from build123d import *

# Parameters (mm, degrees)
F0_R     = 1.6
F1_DEPTH = 2.3
F2_R     = 5.5
F3_DEPTH = 7.7
F5_DEPTH = 26.3
F6_R     = 1
F7_DEPTH = 5.55


with BuildPart() as f1:
    # F0 (on Top) → F1 (new body)
    with BuildSketch(Plane.XY):
        with BuildLine():
            Line((3, 5.765), (-3, 5.765))
            Line((-3, 5.765), (-10.043565, 3.861473))
            ThreePointArc((-10.043565, 3.861473), (-13, 0), (-10.043565, -3.861473))
            Line((-10.043565, -3.861473), (-3, -5.765))
            Line((-3, -5.765), (3, -5.765))
            Line((3, -5.765), (10.043565, -3.861473))
            ThreePointArc((10.043565, -3.861473), (13, 0), (10.043565, 3.861473))
            Line((10.043565, 3.861473), (3, 5.765))
        make_face()
        with Locations((-9, 0)):
            Circle(F0_R, mode=Mode.SUBTRACT)
        with Locations((9, 0)):
            Circle(F0_R, mode=Mode.SUBTRACT)
    extrude(amount=-F1_DEPTH)

    # F2 (on face) → F3 (join)
    with BuildSketch(Plane(origin=(0, 0, -2.3), x_dir=(1, 0, 0), z_dir=(0, 0, -1))):
        Circle(F2_R)
    extrude(amount=F3_DEPTH)

    # F4 (on face) → F5 (join)
    with BuildSketch(Plane(origin=(0, 0, -10), x_dir=(1, 0, 0), z_dir=(0, 0, -1))):
        with BuildLine():
            Line((4, 5.765), (-4, 5.765))
            ThreePointArc((-4, 5.765), (-6.5, 0), (-4, -5.765))
            Line((-4, -5.765), (4, -5.765))
            ThreePointArc((4, -5.765), (6.5, 0), (4, 5.765))
        make_face()
    extrude(amount=F5_DEPTH)

    # F6 (on face) → F7 (join)
    with BuildSketch(Plane(origin=(0, 0, -36.3), x_dir=(1, 0, 0), z_dir=(0, 0, -1))):
        Circle(F6_R)
    extrude(amount=F7_DEPTH)


solid = f1.part
Input: part model. Units: mm. Frame: model coordinates. A direction names the side the tool comes from. Coordinates: 2 decimals unless noted, no trailing zeros. Order: outer loops, then holes, each group sorted by start corner. A loop starts at its lowest first (then second) coordinate and runs counter-clockwise, first axis right, second up. Notation, with made-up numbers: M 33.5,46.25 L 39.5,46.25 A19 ccw 39.5,66.25 Z; hole C -36,4.5 d4. An arc over 180 degrees is marked long. One line per question, with ' | ' between items.
Item 1: Section A-A (x = 9.25). Output: boundary loops of the cut face in (y, z).
Geometry results:
outline: M -4.08,-2.3 L -1.58,-2.3 L -1.58,0 L -4.08,0 Z; M 1.58,-2.3 L 4.08,-2.3 L 4.08,0 L 1.58,0 Z
Item 2: Section B-B (y = 0). Output: boundary loops of the cut face in (x, z), then the cut area to 3 significant figures.
Geometry results:
outline: M -13,-2.3 L -10.6,-2.3 L -10.6,0 L -13,0 Z; M -7.4,-2.3 L -5.5,-2.3 L -5.5,-10 L -6.5,-10 L -6.5,-36.3 L -1,-36.3 L -1,-41.85 L 1,-41.85 L 1,-36.3 L 6.5,-36.3 L 6.5,-10 L 5.5,-10 L 5.5,-2.3 L 7.4,-2.3 L 7.4,0 L -7.4,0 Z; M 10.6,-2.3 L 13,-2.3 L 13,0 L 10.6,0 Z | area: 483 mm^2
Item 3: Draft query along X for faces 6 (the cylindrical face through (0, 1, -39)), 7 (the flat face through (0, -5.765, -23)), 8 (the cylindrical face through (7.4, 0.07, -1.13)), 9 (the cylindrical face through (13, 0, -1)). Return one class per face: released by +X, released by -X, zero draft, split by the parting line, or undercut.
Geometry results:
face 6: split by the parting line | face 7: zero draft | face 8: undercut | face 9: released by +X
Item 4: Section D-D (z = -23.5). Output: boundary loops of the cut face in (x, y) (3 decimals), then the cut area to 3 significant figures.
Geometry results:
outline: M -4,-5.765 L 4,-5.765 A7.897 ccw 4,5.765 L -4,5.765 A7.897 ccw Z | area: 132 mm^2
Item 5: Ray query, line 1 along Z through (x, y) = (-5.5, -3.75); line 2 along Z through (x, y) = (-1.25, 4.75); line 3 along Z through (x, y) = (7.25, 1.25). Return the intervals inside material, ascending.
Geometry results:
line 1: z = -36.3 to -10, -2.3 to 0 | line 2: z = -36.3 to 0 | line 3: z = -2.3 to 0
Item 6: Pin query (flat end, axial travel): pin 1 (1.5 mm diameter, centred on x = -8.5, z = -26.5, fed in from +Y); pin 2 (3 mm diameter, centred on x = 5.5, y = -1.5, fed in from -Z); pin 3 (3 mm diameter, centred on y = -2, z = -24, fed in from -X); pin 4 (2 mm diameter, centred on y = -3, z = -13, fed in from +X). Return the tip coordinate at first contact, or that it passes through.
Geometry results:
pin 1: passes through | pin 2: stops at z = -36.3 | pin 3: stops at x = -6.48 | pin 4: stops at x = 6.24
Item 7: Section C-C (x = 0). Output: boundary loops of the cut face in (y, z) (3 decimals).
Geometry results:
outline: M -5.765,-36.3 L -1,-36.3 L -1,-41.85 L 1,-41.85 L 1,-36.3 L 5.765,-36.3 L 5.765,-10 L 5.5,-10 L 5.5,-2.3 L 5.765,-2.3 L 5.765,0 L -5.765,0 L -5.765,-2.3 L -5.5,-2.3 L -5.5,-10 L -5.765,-10 Z
Item 8: Reachability of faces 1 (the cylindrical face through (-1.19, 5.37, -6.1)), 2 (the flat face through (-6.472, 4.827, -1.134)), 3 (the cylindrical face through (-6.5, -0.1, -23)), 4 (the cylindrical face through (6.5, 0.1, -23)), 5 (the flat face through (-6.57, -4.8, -1.13)) from +Z, -Z, +X, -X, +Y, -Y: full face, straight path, thin tool, end or side. Return the list, or none.
Geometry results:
face 1: none | face 2: +Z, -X, +Y | face 3: -Z, -X | face 4: -Z, +X | face 5: +Z, -X, -Y
